Could you check a few things on this model? Use its own coordinates, in mm. Round coordinates to 2 decimals unless told otherwise and drop trailing zeros. Write each loop counter-clockwise with the first axis right and the second up, starting at its lowest first coordinate (ties: lowest second). Pieces come first, ordered by that corner, then holes. Notation, with made-up numbers: (79.5, 25) -> (137.5, 25) arc R14 ccw to (137.5, 39) -> close; hole circle Ø10 at (89.25, 53.5). An arc over 180 degrees is marked (long way). Answer as CSV lines item,"result". Start each with the question number.
Q1. If I drill on line 1 (Z direction, x = 0, y = -2) (3 decimals); line 2 (Y direction, x = 1.75, z = 21) (3 decimals); line 3 (X direction, y = -1.25, z = 1.5), over which ranges is the centre line in solid material (lowest first)? Write a range as [from, to].
Q2. Imagine slicing it at A-A on z = 14. Please give me the cut outline in (x, y) (3 decimals).
Q3. Imagine slicing it at B-B on z = 26.5. Please give me the cut outline in (x, y) (3 decimals), and give its area (3 significant figures).
Q4. Will these pins go through, and if not, where does the flat tip stop? pin 1 Ø1.5 at (x, y) = (1.5, 2) entering from -Z; pin 2 Ø3 at (x, z) = (1.5, 14.5) entering from -Y (3 decimals); pin 3 Ø4 at (y, z) = (-3.5, 22.5) entering from -X; pin 4 Ø2.5 at (x, z) = (0, 46.04) entering from -Y.
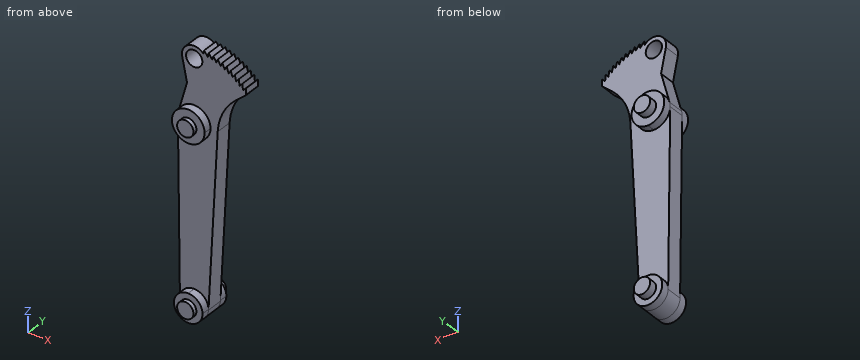
from build123d import *

# Parameters (mm, degrees)
F0_R     = 1.5875
F1_DEPTH = 3.175
F5_DEPTH = 1.5875
F6_R     = 1.5875
F7_DEPTH = 0.79375
F8_R     = 1.5875
F9_DEPTH = 1.5875
F10_R    = 10.31875


# Not quite as in the source:
# - a feature of the source that left no trace in its solid (it failed there, or was rolled back) is left out
# - a pattern or mirror of a feature is missing from the dataset's text; its kind, count and spacing are read off the source's solid


with BuildPart() as f1:
    # F0 (on Front) → F1 (new body)
    with BuildSketch(Plane.XZ):
        with BuildLine():
            Line((-3.1747853497, 34.0943313953), (-2.777937181, -0.0323037791))
            ThreePointArc((-2.777937181, -0.0323037791), (-0.0565749778, -2.7775488812), (2.7743176762, -0.1453958284))
            Line((2.7743176762, -0.1453958284), (4.7932141006, 38.3774428034))
            Line((4.7932141006, 38.3774428034), (10.1004515544, 43.0789965018))
            ThreePointArc((10.1004515544, 43.0789965018), (10.0925772968, 43.0878759884), (10.0846956661, 43.0967489312))
            Line((10.0846956661, 43.0967489312), (10.0430595374, 44.2934156835))
            Line((10.0430595374, 44.2934156835), (9.4851117853, 43.7288509233))
            Line((9.4851117853, 43.7288509233), (9.3663379592, 44.9203356649))
            Line((9.3663379592, 44.9203356649), (8.8459858503, 44.3209420168))
            Line((8.8459858503, 44.3209420168), (8.6505703336, 45.5022785002))
            Line((8.6505703336, 45.5022785002), (8.1699830928, 44.8705546947))
            Line((8.1699830928, 44.8705546947), (7.8987405265, 46.0368182075))
            Line((7.8987405265, 46.0368182075), (7.4599216084, 45.3753977516))
            Line((7.4599216084, 45.3753977516), (7.1139827386, 46.5217264172))
            Line((7.1139827386, 46.5217264172), (6.7187614754, 45.8333666162))
            Line((6.7187614754, 45.8333666162), (6.2995684394, 46.9549816615))
            Line((6.2995684394, 46.9549816615), (5.949592415, 46.2425521248))
            Line((5.949592415, 46.2425521248), (5.4588927295, 47.334777802))
            Line((5.4588927295, 47.334777802), (5.1556209112, 46.6012484796))
            Line((5.1556209112, 46.6012484796), (4.5954601871, 47.6595315582))
            Line((4.5954601871, 47.6595315582), (4.3401568434, 46.9079603605))
            Line((4.3401568434, 46.9079603605), (3.7128702582, 47.9278891087))
            Line((3.7128702582, 47.9278891087), (3.5065996883, 47.1614091582))
            Line((3.5065996883, 47.1614091582), (2.8148022515, 48.1387317342))
            Line((2.8148022515, 48.1387317342), (2.6584243486, 47.3605383046))
            Line((2.6584243486, 47.3605383046), (1.905, 48.2911804818))
            Line((1.905, 48.2911804818), (1.8099761367, 47.5848648397))
            ThreePointArc((1.8099761367, 47.5848648397), (-1.0450737271, 48.1771664384), (-2.33313898, 45.56125))
            Line((-2.33313898, 45.56125), (-1.3985654512, 40.9827934547))
            Line((-1.3985654512, 40.9827934547), (-3.0600295024, 34.9779166667))
            ThreePointArc((-3.0600295024, 34.9779166667), (-3.1485567794, 34.5401695607), (-3.1747853497, 34.0943313953))
        make_face()
        with Locations((0, 46.0375)):
            Circle(F0_R, mode=Mode.SUBTRACT)
    extrude(amount=F1_DEPTH)

    # F4 (on face) → F5 (join)
    with BuildSketch(Plane.XZ.offset(3.175)):
        with BuildLine():
            ThreePointArc((0, 2.778125), (-1.9644310265, -1.9644310265), (2.778125, 0))
            ThreePointArc((2.778125, 0), (1.9644310265, 1.9644310265), (0, 2.778125))
        make_face()
        with BuildLine():
            ThreePointArc((3.175, 34.13125), (-2.2450640303, 36.3763140303), (0, 30.95625))
            ThreePointArc((0, 30.95625), (2.2450640303, 31.8861859697), (3.175, 34.13125))
        make_face()
    f5 = extrude(amount=F5_DEPTH)

    # F5_copies: F5 across plane
    add(f5.mirror(Plane.ZX.offset(-1.5875)))

    # F6 (on face) → F7 (join)
    with BuildSketch(Plane.XZ.offset(4.7625)):
        Circle(F6_R)
        with Locations((0, 34.13125)):
            Circle(F6_R)
    extrude(amount=F7_DEPTH)

    # F8 (on face) → F9 (join)
    with BuildSketch(Plane(origin=(0, 1.5875, 0), x_dir=(-1, 0, 0), z_dir=(0, 1, 0))):
        Circle(F8_R)
        with Locations((0, 34.13125)):
            Circle(F8_R)
    extrude(amount=F9_DEPTH)

    # F10
    f10_edges = [f1.edges().sort_by_distance(p)[0] for p in [
        (4.793214, -1.5875, 38.377443),
    ]]
    fillet(f10_edges, radius=F10_R)


solid = f1.part
Checks:
1,line 1,"[-2.778, 44.45], [47.625, 48.419]"
1,line 2,"[-3.175, 0]"
1,line 3,"[-2.8, 2.86]"
2,outline,"(-2.941, -3.175) -> (3.516, -3.175) -> (3.516, 0) -> (-2.941, 0) -> close"
3,outline,"(-3.086, -3.175) -> (4.171, -3.175) -> (4.171, 0) -> (-3.086, 0) -> close"
3,area,"23.0 mm^2"
4,pin 1,"z = -2.64"
4,pin 2,"y = -3.175"
4,pin 3,"x = -3.06"
4,pin 4,"through"
